Source: three-view drawing plus pictorial views. Frame: mm from the lowest corner of the part. A direction names the side the tool comes from. Round coordinates to 2 decimals unless told otherwise and drop trailing zeros. Write each loop counter-clockwise with the first axis right and the second up, starting at its lowest first coordinate (ties: lowest second). Pieces come first, ordered by that corner, then holes.
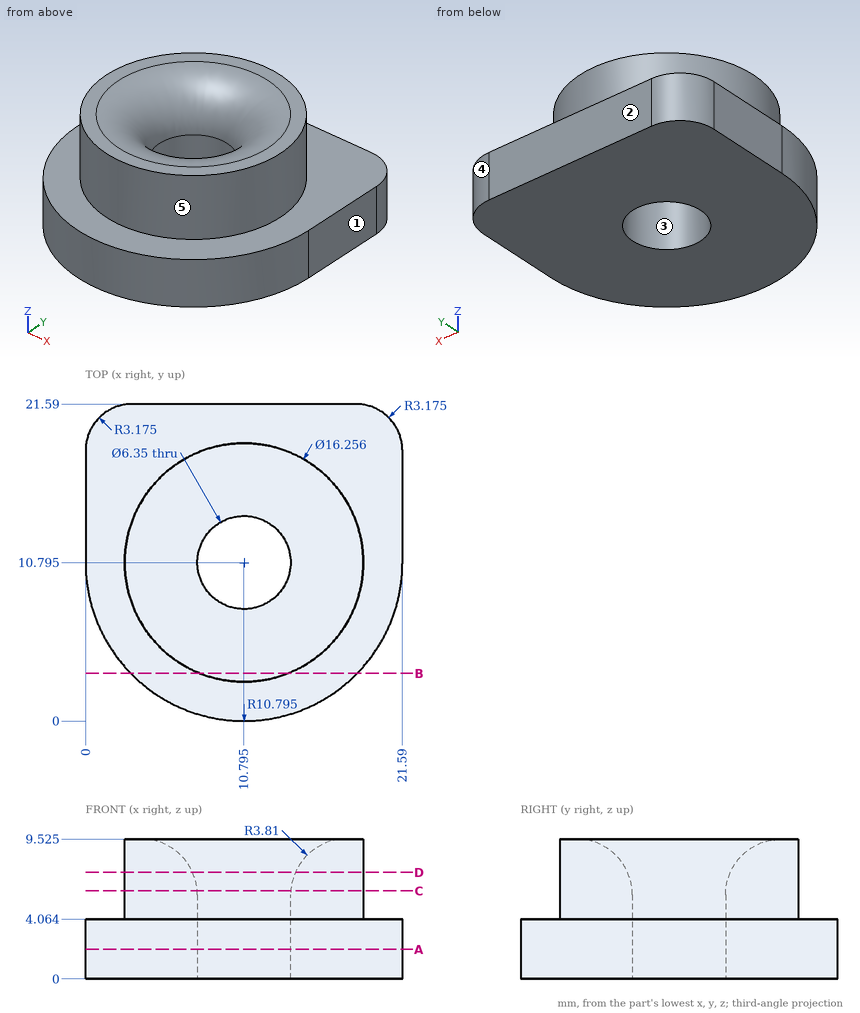
1) Section D-D on z = 7.25. Output: boundary loops of the cut face in (x, y) (3 decimals), plus the area to 3 significant figures.
2) Reachability of the marked faces 4 and 5 from +Z, -Z, +X, -X, +Y, -Y: full face, straight path, thin tool, end or side. Return the list, or none.
3) Section A-A on z = 2. Output: boundary loops of the cut face in (x, y) (3 decimals), plus the area to 3 significant figures.
4) First-contact query: P1, Ø6.5, axis at x = 9, y = 8.5, coming from the +Z side; P2, Ø10, axis at x = 2.5, y = 8, coming from the +Z side (3 decimals); P3, Ø4, axis at x = 10.795, y = 10.795, coming from the +Z side; P4, Ø1.5, axis at y = 15.5, z = 5.5, coming from the -X side. Flat tips, straight axial feed; report the tip coordinate or a pass-through.
5) Draft query along Y for the marked faces 1, 2 and 3. Return one class per face: pulls with the +Y half, pulls with the -Y half, needs draft (parallel to the pull), parting line crosses it, or undercut.
6) Section C-C on z = 6. Output: boundary loops of the cut face in (x, y) (3 decimals), plus the area to 3 significant figures.
7) Section B-B on y = 3.25. Output: boundary loops of the cut face in (x, z) (3 decimals), plus the area to 3 significant figures.
8) Line query: probe 1 along X at (y, z) = (10.75, 4.5); probe 2 along Z at (x, y) = (4.25, 8.75); probe 3 along Y at (x, z) = (9.5, 3). Output: solid intervals per line, ascending.
Filled in:
1. outline: circle Ø16.256 at (10.795, 10.795); hole circle Ø6.996 at (10.795, 10.795)
1. area: 169 mm2
2. face 4: +Z, -Z, +X, +Y
2. face 5: +Z
3. outline: (0, 10.795) arc R10.795 ccw to (21.59, 10.795) - (21.59, 18.415) arc R3.175 ccw to (18.415, 21.59) - (3.175, 21.59) arc R3.175 ccw to (0, 18.415) - close; hole circle Ø6.35 at (10.795, 10.795)
3. area: 380 mm2
4. P1: stops at z = 9.44
4. P2: stops at z = 9.525
4. P3: passes through
4. P4: stops at x = 3.69
5. face 1: needs draft
5. face 2: pulls with the +Y half
5. face 3: undercut
6. outline: circle Ø16.256 at (10.795, 10.795); hole circle Ø6.371 at (10.795, 10.795)
6. area: 176 mm2
7. outline: (3.075, 0) - (18.515, 0) - (18.515, 4.064) - (13.818, 4.064) - (13.818, 9.525) - (7.772, 9.525) - (7.772, 4.064) - (3.075, 4.064) - close
7. area: 95.8 mm2
8. probe 1: x = 2.67 to 7.62, 13.97 to 18.92
8. probe 2: z = 0 to 9.52
8. probe 3: y = 0.08 to 7.9, 13.69 to 21.59
